CAD build for the part. Positions are in the model's coordinates, mm. Round coordinates to 2 decimals unless told otherwise and drop trailing zeros. Order: outer loops, then holes, each group sorted by start corner. A loop starts at its lowest first (then second) coordinate and runs counter-clockwise, first axis right, second up.
```python
from build123d import *

# Parameters (mm, degrees)
F0_W     = 12.73
F0_H     = 120
F1_DEPTH = 1.3
F2_W     = 7.3
F2_H     = 13
F3_DEPTH = 1.3


with BuildPart() as f1:
    # F0 (on Top) → F1 (new body)
    with BuildSketch(Plane.XY):
        with Locations((-18.500336, -0.08574)):
            Rectangle(F0_W, F0_H)
    extrude(amount=F1_DEPTH)

    # F2 (on Top) → F3 (join)
    with BuildSketch(Plane.XY):
        with Locations((-18.497536, -66.319867)):
            Rectangle(F2_W, F2_H)
    extrude(amount=F3_DEPTH)


solid = f1.part
```
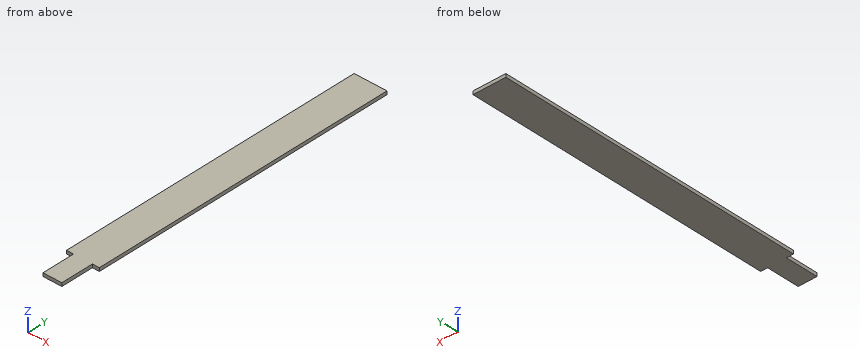
1. Cut at A-A, the plane z = 1. Write the cut outline in (x, y).
2. Cut at B-B, the plane x = -23.25. Write the cut outline in (y, z).
3. Drill centre lines: line 1 (Y direction, x = -22.5, z = 1.15); line 2 (X direction, y = -64.5, z = 0.6). Where is each one in solid material? Low to high.
4. Pin check, flat tip, straight feed: P1, Ø0.6, axis at y = -67, z = 1, coming from the -X side. Stop position of the tip, or through.
Outcome:
1. outline: (-24.87, -60.09) - (-22.15, -60.09) - (-22.15, -72.82) - (-14.85, -72.82) - (-14.85, -60.09) - (-12.14, -60.09) - (-12.14, 59.91) - (-24.87, 59.91) - close
2. outline: (-60.09, 0) - (59.91, 0) - (59.91, 1.3) - (-60.09, 1.3) - close
3. line 1: y = -60.09 to 59.91
3. line 2: x = -22.15 to -14.85
4. P1: stops at x = -22.15
